```python
from build123d import *

# Parameters (mm, degrees)
CONNECTOR_M5X0_8_TAPPED_HOLE_D        = 4.2
SET_SCREW_1_M3X0_5_TAPPED_HOLE_REACH  = 16.767
SET_SCREW_1_M3X0_5_TAPPED_HOLE_BORE_R = 1.25


with BuildPart() as part:
    # Body Sketch → Body Revolve (revolve)
    with BuildSketch(Plane(origin=(0, 0, 0), x_dir=(-1, 0, 0), z_dir=(0, 1, 0))):
        Polygon((1, 10.5), (4, 10.5), (4, 8), (5.4, 4), (5.4, 0), (2.5, 0), (2.5, 5), (1, 5), align=None)
    revolve(axis=Axis((0, 0, 0), (0, 0, 1)))

    # Connector M5x0.8 Tapped Hole (through all)
    with Locations(Plane.XY.offset(10.5)):
        with Locations((0, 0)):
            Hole(CONNECTOR_M5X0_8_TAPPED_HOLE_D / 2)

    # Set Screw 1 M3x0.5 Tapped Hole bore (on position points) → Set Screw 1 M3x0.5 Tapped Hole (cut, up to next)
    with BuildSketch(Plane(origin=(5.4, 0, 2), x_dir=(0, 1, 0), z_dir=(1, 0, 0)), mode=Mode.PRIVATE) as set_screw_1_m3x0_5_tapped_hole_sk1:
        Circle(SET_SCREW_1_M3X0_5_TAPPED_HOLE_BORE_R)
    set_screw_1_m3x0_5_tapped_hole_tool1 = extrude(set_screw_1_m3x0_5_tapped_hole_sk1.sketch, amount=-SET_SCREW_1_M3X0_5_TAPPED_HOLE_REACH, mode=Mode.PRIVATE) & part.part
    add(set_screw_1_m3x0_5_tapped_hole_tool1.solids().sort_by_distance((5.4, 0, 2))[0], mode=Mode.SUBTRACT)


solid = part.part
```
CAD build for the part. Positions are in the model's coordinates, mm. A direction names the side the tool comes from. Give positions to 0.01 mm unless a question says otherwise; leave off trailing zeros. Loops run counter-clockwise (first coordinate to the right, second up) from the corner with the lowest first, then second, coordinate; pieces in that order, holes last. Notation, with made-up numbers: (70, 34.25) -> (86, 34.25) arc R37 cw to (86, 73.25) -> close; hole circle Ø9 at (73.25, 85.25). An arc over 180 degrees is marked (long way). Use a Markdown table: item, result.
1. Flat gauge pins, fed straight in: pin 1 (2.5 mm diameter, centred on x = 0, y = 0, fed in from +Z); pin 2 (2 mm diameter, centred on y = 0, z = 2, fed in from +X); pin 3 (2.5 mm diameter, centred on x = 1, y = -0.5, fed in from -Z); pin 4 (6 mm diameter, centred on x = -1, z = 9, fed in from -Y). Where does each tip first touch, or does it go through?
Check result:
| item | result |
|---|---|
| pin 1 | passes through |
| pin 2 | stops at x = -2.29 |
| pin 3 | stops at z = 5 |
| pin 4 | stops at y = -4.66 |
2. Which spindle directions (+Z, -Z, +X, -X, +Y, -Y) get a long thin tool onto all of the face, cutting with end or side? Do faces 1 (the cylindrical face through (-2.003, 0.631, 7.712)), 2 (the cylindrical face through (0.867, 3.905, 9.232)), 3 (the cylindrical face through (-2.385, -0.751, 2.535)). Say none if no direction does.
Check result:
| item | result |
|---|---|
| face 1 | +Z, -Z |
| face 2 | +Z |
| face 3 | -Z |
3. Slice it at B-B (y = 0). List the corners of the cut face in (x, z).
Check result:
| item | result |
|---|---|
| outline | (-5.4, 0) -> (-2.5, 0) -> (-2.5, 5) -> (-2.1, 5) -> (-2.1, 10.5) -> (-4, 10.5) -> (-4, 8) -> (-5.4, 4) -> close; (2.1, 5) -> (2.5, 5) -> (2.5, 3.25) -> (5.4, 3.25) -> (5.4, 4) -> (4, 8) -> (4, 10.5) -> (2.1, 10.5) -> close; (2.5, 0) -> (5.4, 0) -> (5.4, 0.75) -> (2.5, 0.75) -> close |
4. Slice it at C-C (z = 9.5). List the corners of the cut face in (x, y), plus the area to 3 significant figures.
Check result:
| item | result |
|---|---|
| outline | circle Ø8 at (0, 0); hole circle Ø4.2 at (0, 0) |
| area | 36.4 mm^2 |
5. Wall check: L1, parallel to Z at x = 0.5, y = 2.25; L2, parallel to Y at x = 0, z = 8; L3, parallel to Y at x = 3.5, z = 2. Give the ranges that are in metal, low to high. Write a range as [from, to].
Check result:
| item | result |
|---|---|
| L1 | z = [5, 10.5] |
| L2 | y = [-4, -2.1], [2.1, 4] |
| L3 | y = [-4.11, -1.25], [1.25, 4.11] |
6. Mould opens along Y. For faces 4 (the flat face through (2, 2, 10.5)), 5 (the cylindrical face through (-5.15, -1.62, 1.97)), 6 (the cylindrical face through (3.81, -1.25, 2.05)) say: pulls with the +Y half, pulls with the -Y half, needs draft (parallel to the pull), parting line crosses it, or undercut.
Check result:
| item | result |
|---|---|
| face 4 | needs draft |
| face 5 | parting line crosses it |
| face 6 | undercut |
7. Slice it at A-A (x = 0). List the corners of the cut face in (y, z), plus the area to 3 significant figures.
Check result:
| item | result |
|---|---|
| outline | (-5.4, 0) -> (-2.5, 0) -> (-2.5, 5) -> (-2.1, 5) -> (-2.1, 10.5) -> (-4, 10.5) -> (-4, 8) -> (-5.4, 4) -> close; (2.1, 5) -> (2.5, 5) -> (2.5, 0) -> (5.4, 0) -> (5.4, 4) -> (4, 8) -> (4, 10.5) -> (2.1, 10.5) -> close |
| area | 52.7 mm^2 |
8. Slice it at D-D (z = 3.5). List the corners of the cut face in (x, y), plus the area to 3 significant figures.
Check result:
| item | result |
|---|---|
| outline | circle Ø10.8 at (0, 0); hole circle Ø5 at (0, 0) |
| area | 72.0 mm^2 |
